Build history of the part. All positions in model axes, mm. A direction names the side the tool comes from. Coordinates: 2 decimals unless noted, no trailing zeros. Loops run counter-clockwise (first coordinate to the right, second up) from the corner with the lowest first, then second, coordinate; pieces in that order, holes last. Notation, with made-up numbers: (-4, 49.25) - (20, 49.25) arc R22 ccw to (20, 77.25) - close; hole circle Ø3 at (11.25, -33.75). An arc over 180 degrees is marked (long way). One line per item, written item: value.
Autodesk Fusion 360 part; units mm, degrees
sketch "Sketch1" plane through (0, 0, 0) normal (0, 0, 1) x (1, 0, 0)
  circle A0 centre (0, 0) radius 8.295
  dimension "d1" = 16.59
sketch "Sketch3" plane through (0, 0, 0) normal (0, 0, 1) x (1, 0, 0)
ref_plane "WorkPlane1" through (0, 0, 106.36) normal (0, 0, 1) x (1, 0, 0)
sketch "Sketch4" plane through (0, 0, 106.36) normal (0, 0, 1) x (1, 0, 0)
  circle A0 centre (0, 0) radius 5.07
  dimension "d4" = 10.14
loft "Loft1" add profiles "Sketch4", "Sketch1" section 1 section 2
sketch "Sketch5" plane through (0, 0, 106.36) normal (0, 0, 1) x (-1, 0, 0)
  circle A0 centre (0, 0) radius 5.07
ref_plane "WorkPlane3" through (0, 0, 140.11) normal (0, 0, 1) x (-1, 0, 0)
sketch "Sketch6" plane through (0, 0, 140.11) normal (0, 0, 1) x (1, 0, 0)
  circle A0 centre (0, 0) radius 1.465
  dimension "d6" = 2.93
loft "Loft2" add profiles "Sketch5", "Sketch6" section 1 section 2
sketch "Sketch7" plane through (0, 0, 0) normal (0, 0, -1) x (1, 0, 0)
  circle A0 centre (0, 0) radius 8.295
ref_plane "WorkPlane4" through (0, 0, -15.77) normal (0, 0, -1) x (1, 0, 0)
sketch "Sketch8" plane through (0, 0, -15.77) normal (0, 0, -1) x (1, 0, 0)
  circle A0 centre (0, 0) radius 9.305
  dimension "d8" = 18.61
extrude "Extrude1" add sketch "Sketch7" along normal blind 15.77
sketch "Sketch9" plane through (0, 0, 0) normal (0, 0, 1) x (1, 0, 0)
extrude "Extrude2" add sketch "Sketch8" against normal blind 15.77
sketch "Sketch10" plane through (0, 0, 0) normal (0, 0, 1) x (-1, 0, 0)
  circle A0 centre (0, 0) radius 9.305
  circle A1 centre (0, 0) radius 8.295
  line L0 (-0.4459, 8.295) -> (0.4341, 8.295)
  line L1 (0.4341, 8.295) -> (0.4341, 10.295)
  line L2 (0.4341, 10.295) -> (-0.4459, 10.295)
  line L3 (-0.4459, 10.295) -> (-0.4459, 8.295)
  line L4 (-0.0059, 10.295) -> (-0.0059, 8.295)
  line L5 (-0.0059, 8.295) -> (-0.0059, 9.305)
  line L6 (-4.3517, 9.3407) -> (-3.5863, 7.493)
  line L7 (-3.5386, 9.6775) -> (-4.3517, 9.3407)
  line L8 (-3.5863, 7.493) -> (-2.7733, 7.8297)
  line L9 (-2.7733, 7.8297) -> (-3.5386, 9.6775)
  line L10 (-7.5949, 6.9644) -> (-6.1807, 5.5502)
  line L11 (-6.9727, 7.5866) -> (-7.5949, 6.9644)
  line L12 (-6.1807, 5.5502) -> (-5.5585, 6.1724)
  line L13 (-5.5585, 6.1724) -> (-6.9727, 7.5866)
  line L14 (-9.682, 3.5278) -> (-7.8342, 2.7624)
  line L15 (-9.3452, 4.3408) -> (-9.682, 3.5278)
  line L16 (-7.8342, 2.7624) -> (-7.4974, 3.5754)
  line L17 (-7.4974, 3.5754) -> (-9.3452, 4.3408)
  line L18 (-10.295, -0.4459) -> (-8.295, -0.4459)
  line L19 (-10.295, 0.4341) -> (-10.295, -0.4459)
  line L20 (-8.295, -0.4459) -> (-8.295, 0.4341)
  line L21 (-8.295, 0.4341) -> (-10.295, 0.4341)
  line L22 (-9.3407, -4.3517) -> (-7.493, -3.5863)
  line L23 (-9.6775, -3.5386) -> (-9.3407, -4.3517)
  line L24 (-7.493, -3.5863) -> (-7.8297, -2.7733)
  line L25 (-7.8297, -2.7733) -> (-9.6775, -3.5386)
  line L26 (-6.9644, -7.5949) -> (-5.5502, -6.1807)
  line L27 (-7.5866, -6.9727) -> (-6.9644, -7.5949)
  line L28 (-5.5502, -6.1807) -> (-6.1724, -5.5585)
  line L29 (-6.1724, -5.5585) -> (-7.5866, -6.9727)
  line L30 (-3.5278, -9.682) -> (-2.7624, -7.8342)
  line L31 (-4.3408, -9.3452) -> (-3.5278, -9.682)
  line L32 (-2.7624, -7.8342) -> (-3.5754, -7.4974)
  line L33 (-3.5754, -7.4974) -> (-4.3408, -9.3452)
  line L34 (0.4459, -10.295) -> (0.4459, -8.295)
  line L35 (-0.4341, -10.295) -> (0.4459, -10.295)
  line L36 (0.4459, -8.295) -> (-0.4341, -8.295)
  line L37 (-0.4341, -8.295) -> (-0.4341, -10.295)
  line L38 (4.3517, -9.3407) -> (3.5863, -7.493)
  line L39 (3.5386, -9.6775) -> (4.3517, -9.3407)
  line L40 (3.5863, -7.493) -> (2.7733, -7.8297)
  line L41 (2.7733, -7.8297) -> (3.5386, -9.6775)
  line L42 (7.5949, -6.9644) -> (6.1807, -5.5502)
  line L43 (6.9727, -7.5866) -> (7.5949, -6.9644)
  line L44 (6.1807, -5.5502) -> (5.5585, -6.1724)
  line L45 (5.5585, -6.1724) -> (6.9727, -7.5866)
  line L46 (9.682, -3.5278) -> (7.8342, -2.7624)
  line L47 (9.3452, -4.3408) -> (9.682, -3.5278)
  line L48 (7.8342, -2.7624) -> (7.4974, -3.5754)
  line L49 (7.4974, -3.5754) -> (9.3452, -4.3408)
  line L50 (10.295, 0.4459) -> (8.295, 0.4459)
  line L51 (10.295, -0.4341) -> (10.295, 0.4459)
  line L52 (8.295, 0.4459) -> (8.295, -0.4341)
  line L53 (8.295, -0.4341) -> (10.295, -0.4341)
  line L54 (9.3407, 4.3517) -> (7.493, 3.5863)
  line L55 (9.6775, 3.5386) -> (9.3407, 4.3517)
  line L56 (7.493, 3.5863) -> (7.8297, 2.7733)
  line L57 (7.8297, 2.7733) -> (9.6775, 3.5386)
  line L58 (6.9644, 7.5949) -> (5.5502, 6.1807)
  line L59 (7.5866, 6.9727) -> (6.9644, 7.5949)
  line L60 (5.5502, 6.1807) -> (6.1724, 5.5585)
  line L61 (6.1724, 5.5585) -> (7.5866, 6.9727)
  line L62 (3.5278, 9.682) -> (2.7624, 7.8342)
  line L63 (4.3408, 9.3452) -> (3.5278, 9.682)
  line L64 (2.7624, 7.8342) -> (3.5754, 7.4974)
  line L65 (3.5754, 7.4974) -> (4.3408, 9.3452)
  dimension "d14" = 0.88
  dimension "d15" = 2
  dimension "d17" = 360
extrude "Extrude3" cut sketch "Sketch10" against normal blind 15 contours A0 A1 L50 L52 L56 L57 | A0 A1 L46 L48 L52 L53 | A0 A1 L54 L56 L60 L61 | A0 A1 L42 L44 L48 L49 | A0 A1 L58 L60 L64 L65 | A0 A1 L38 L40 L44 L45 | A0 A1 L0 L3 L8 L9 | A0 A1 L0 L1 L62 L64 | A0 A1 L34 L36 L40 L41 | A0 A1 L30 L32 L36 L37 | A0 A1 L6 L8 L12 L13 | A0 A1 L26 L28 L32 L33 | A0 A1 L10 L12 L16 L17 | A0 A1 L22 L24 L28 L29 | A0 A1 L14 L16 L20 L21 | A0 A1 L18 L20 L24 L25
sketch "Sketch11" plane through (0, 0, -15.77) normal (0, 0, -1) x (1, 0, 0)
  circle A0 centre (0, 0) radius 9.305
  circle A1 centre (0, 0) radius 7.445
  dimension "d20" = 14.89
extrude "Extrude4" cut sketch "Sketch11" against normal blind 16 contours A1
ref_plane "WorkPlane2" through (0, 0, 106.36) normal (0, 0, 1) x (1, 0, 0)
Item 1: Cut at A-A, the plane z = 77. Write the cut outline in (x, y).
Check result:
outline: circle Ø11.92 at (0, 0)
Item 2: Pull direction Z, two halves, no side cores. Call faces 3 (the face through (-1.64, -8.13, -7.4)), 4 (the face through (-1.6, 8.14, -7.4)), 5 (the face through (6.88, 2.85, -7.88)), 6 (the face through (6.4, -2, 52.4)): released by +Z, released by -Z, zero draft, split by the parting line, or undercut.
Check result:
face 3: undercut
face 4: undercut
face 5: zero draft
face 6: released by +Z
Item 3: Cut at B-B, the plane z = 108. Write the cut outline in (x, y), then the cut area to 3 significant figures.
Check result:
outline: circle Ø9.79 at (0, 0)
area: 75.3 mm^2
Item 4: Probe probe 1 along Z at (x, y) = (0.5, -1.25); probe 2 along Y at (x, z) = (5.75, 62.5); probe 3 along Y at (x, z) = (-4.75, -7.5). List the from-to ranges inside material, lowest first. Write a range as from..to.
Check result:
probe 1: z = 0.23..140.11
probe 2: y = -2.81..2.81
probe 3: y = -6.8..-5.73, 5.73..6.8
Item 5: Drop flat-ended pins along their axis: P1, Ø4, axis at y = 2.5, z = 49, coming from the -X side; P2, Ø4, axis at x = 5.5, z = 67, coming from the +Y side; P3, Ø0.6, axis at x = 8, y = 3.5, coming from the +Z side. Give the stop position or say it passes through.
Check result:
P1: stops at x = -6.8
P2: stops at y = 5.2
P3: stops at z = 0
Item 6: Tool access for faces 1 (the face through (-8.13, 1.64, -7.4)), 2 (the face through (0, 0, 0.23)): list every direction of +Z, -Z, +X, -X, +Y, -Y with a clear straight run to the whole face (end or side of a thin tool).
Check result:
face 1: none
face 2: -Z
